```python
from build123d import *


with BuildPart() as part:
    # Sketch2 → Revolve1 (revolve)
    with BuildSketch(Plane(origin=(0, 0, 0), x_dir=(1, 0, 0), z_dir=(0, 1, 0))):
        with BuildLine():
            Line((-340.36, 635), (340.36, 635))
            ThreePointArc((340.36, 635), (378.077075708, 650.622924292), (393.7, 688.34))
            Line((393.7, 688.34), (393.7, 939.8))
            Line((393.7, 939.8), (227.184506514, 939.8))
            ThreePointArc((227.184506514, 939.8), (0, 838.2), (-227.184506514, 939.8))
            Line((-227.184506514, 939.8), (-393.7, 939.8))
            Line((-393.7, 939.8), (-393.7, 688.34))
            ThreePointArc((-393.7, 688.34), (-378.077075708, 650.622924292), (-340.36, 635))
        make_face()
    revolve(axis=Axis((-586.613, 0, 0), (1, 0, 0)))


solid = part.part
```
Input: part model. Units: mm. Frame: model coordinates. Round coordinates to 2 decimals unless told otherwise and drop trailing zeros. Loops run counter-clockwise (first coordinate to the right, second up) from the corner with the lowest first, then second, coordinate; pieces in that order, holes last. Notation, with made-up numbers: (-7, -19) -> (21, -19) arc R27 cw to (21, 0) -> close; hole circle Ø4 at (-19.75, 10). An arc over 180 degrees is marked (long way). Write each question's results on one line, items separated by ' | '.
1. Section D-D (x = 74). Return loops of the section in (y, z), and give its area (3 significant figures).
Geometry results:
outline: circle Ø1694.64 at (0, 0); hole circle Ø1270 at (0, 0) | area: 989,000 mm2
2. Ray query, line 1 (Y direction, x = -42, z = 0); line 2 (Y direction, x = -63, z = 0); line 3 (Z direction, x = -188.5, y = 553.5). Return the intervals inside material, ascending. Write a range as from..to.
Geometry results:
line 1: -841.11..-635, 635..841.11 | line 2: -844.78..-635, 635..844.78 | line 3: -714.08..-311.23, 311.23..714.08
3. Section C-C (x = -175.5). Return loops of the section in (y, z), and give its area (3 significant figures).
Geometry results:
outline: circle Ø1787.59 at (0, 0); hole circle Ø1270 at (0, 0) | area: 1,240,000 mm2
4. First-contact query: P1, Ø10, axis at x = -18, z = 106.5, coming from the +Y side; P2, Ø8, axis at x = -256.5, y = -83, coming from the -Z side; P3, Ø6, axis at x = -44.5, y = -565, coming from the +Z side. Flat tips, straight axial feed; report the tip coordinate or a pass-through.
Geometry results:
P1: y = 832.65 | P2: z = -936.47 | P3: z = 626.34
5. Mould query, pull axis Z, two halves, no side actions, for faces 1 (the face through (-393.7, 492, 492)), 2 (the face through (4.765, 190.737, -605.677)), 3 (the face through (-311.608, -571.854, 745.793)). Classes: +Z half, -Z half, draft (parallel to the pull), parting line (faces both ways), or undercut.
Geometry results:
face 1: draft | face 2: undercut | face 3: parting line
6. Section A-A (z = 0). Return loops of the section in (x, y).
Geometry results:
outline: (-393.7, -939.8) -> (-227.18, -939.8) arc R304.8 cw to (227.18, -939.8) -> (393.7, -939.8) -> (393.7, -688.34) arc R53.34 ccw to (340.36, -635) -> (-340.36, -635) arc R53.34 ccw to (-393.7, -688.34) -> close; (-393.7, 688.34) arc R53.34 ccw to (-340.36, 635) -> (340.36, 635) arc R53.34 ccw to (393.7, 688.34) -> (393.7, 939.8) -> (227.18, 939.8) arc R304.8 cw to (-227.18, 939.8) -> (-393.7, 939.8) -> close
